```python
from build123d import *

# Parameters (mm, degrees)
F0_W     = 120
F0_H     = 22
F1_DEPTH = 10
F3_D     = 3.4544
F5_D     = 4.4958
F6_W     = 2.5
F6_H     = 7


with BuildPart() as f1:
    # F0 (on Top) → F1 (new body)
    with BuildSketch(Plane.XY):
        Rectangle(F0_W, F0_H)
    extrude(amount=F1_DEPTH)

    # F3 (through all)
    with Locations(Plane.XY.offset(10)):
        with Locations((-50, 0)):
            Hole(F3_D / 2)

    # F5 (through all)
    with Locations(Plane.XY.offset(10)):
        with Locations((-36.5, 0), (50, 0)):
            Hole(F5_D / 2)

    # F6 (on Front) → F7 (revolve, cut)
    with BuildSketch(Plane.XZ):
        with Locations((-34.25, 6.5)):
            Rectangle(F6_W, F6_H)
    revolve(axis=Axis((-36.5, 0, 5), (0, 0, -1)), mode=Mode.SUBTRACT)


solid = f1.part
```
The listing builds one solid part. Answer for the finished solid, in the listing's coordinates (mm). A direction names the side the tool comes from. Give positions to 0.01 mm unless a question says otherwise; leave off trailing zeros. Loops run counter-clockwise (first coordinate to the right, second up) from the corner with the lowest first, then second, coordinate; pieces in that order, holes last. Notation, with made-up numbers: (74, -6.75) - (100, -6.75) arc R23 cw to (100, 29.25) - close; hole circle Ø2 at (-25.5, 75). An arc over 180 degrees is marked (long way). Return JSON: item names as keys, results as strings. Group by question number.
1. Find section D-D (x = -50). Write down the section's boundary in (y, z), then the cut area to 3 significant figures.
2. Find section B-B (z = 5). Write down the section's boundary in (x, y).
3. Determine the mould class of faces 1 (the cylindrical face through (-40, 0, 7)), 2 (the flat face through (-1, 11, 5)), 3 (the flat face through (60, 0, 5)) for opening direction X: pulls with the +X half, pulls with the -X half, needs draft (parallel to the pull), parting line crosses it, or undercut.
4. Straight lines are drawn through the part: line 1 (Y direction, x = -36.5, z = 8.5); line 2 (Y direction, x = -34, z = 8). For each, find the intervals that lie inside material, in ascending order. Write a range as [from, to].
5. Find section C-C (x = -36.5). Write down the section's boundary in (y, z).
6. Which of the six approach directions +Z, -Z, +X, -X, +Y, -Y give full straight-line access (tool end or side, diameter ignored) to faces 4 (the flat face through (-39, 0, 3)), 5 (the flat face through (-60, 0, 5))?
7. Find section A-A (y = 0). Write down the section's boundary in (x, z), then the cut area to 3 significant figures.
8. Given pin 1 Ø2 at (x, y) = (-38, 0.5) entering from +Z, flat-ended and moving along its own axis, determine where the tip first touches the part or whether it passes through.
Verdict:
{
 "1": {"outline": "(-11, 0) - (-1.73, 0) - (-1.73, 10) - (-11, 10) - close; (1.73, 0) - (11, 0) - (11, 10) - (1.73, 10) - close", "area": "185 mm^2"},
 "2": {"outline": "(-60, -11) - (60, -11) - (60, 11) - (-60, 11) - close; hole circle Ø3.45 at (-50, 0); hole circle Ø7 at (-36.5, 0); hole circle Ø4.5 at (50, 0)"},
 "3": {"face 1": "undercut", "face 2": "needs draft", "face 3": "pulls with the +X half"},
 "4": {"line 1": "y = [-11, -3.5], [3.5, 11]", "line 2": "y = [-11, -2.45], [2.45, 11]"},
 "5": {"outline": "(-11, 0) - (-2.25, 0) - (-2.25, 3) - (-3.5, 3) - (-3.5, 10) - (-11, 10) - close; (2.25, 0) - (11, 0) - (11, 10) - (3.5, 10) - (3.5, 3) - (2.25, 3) - close"},
 "6": {"face 4": "+Z", "face 5": "+Z, -Z, -X, +Y, -Y"},
 "7": {"outline": "(-60, 0) - (-51.73, 0) - (-51.73, 10) - (-60, 10) - close; (-48.27, 0) - (-38.75, 0) - (-38.75, 3) - (-40, 3) - (-40, 10) - (-48.27, 10) - close; (-34.25, 0) - (47.75, 0) - (47.75, 10) - (-33, 10) - (-33, 3) - (-34.25, 3) - close; (52.25, 0) - (60, 0) - (60, 10) - (52.25, 10) - close", "area": "1,060 mm^2"},
 "8": {"pin 1": "stops at z = 3"}
}
